```python
from build123d import *

# Parameters (mm, degrees)
F0_W     = 2.5
F0_H     = 84.828298
F0_H_2   = 45.171702
F1_DEPTH = 6
F3_COUNT = 2
F3_ANGLE = 180


with BuildPart() as f1:
    # F0 (on Top) → F1 (new body)
    with BuildSketch(Plane.XY):
        with BuildLine():
            Line((192.326957, -18.864548), (-57.173043, -18.864548))
            Line((-57.173043, -18.864548), (-57.173043, -69.03625))
            ThreePointArc((-57.173043, -69.03625), (-55.427418, -65.103617), (-51.781147, -62.819426))
            Line((-51.781147, -62.819426), (170.496624, -45.052804))
            ThreePointArc((170.496624, -45.052804), (186.918172, -36.548754), (192.326957, -18.864548))
        make_face()
        Polygon((-60.173043, -18.864548), (-57.173043, -18.864548), (-57.173043, 70.96375), (-60.173043, 70.96375), (-60.173043, 65.96375), align=None)
        with Locations((-61.423043, 23.549601)):
            Rectangle(F0_W, F0_H)
        Polygon((-57.173043, -69.03625), (-57.173043, -18.864548), (-60.173043, -18.864548), (-60.173043, -64.03625), (-60.173043, -69.03625), align=None)
        with Locations((-61.423043, -41.450399)):
            Rectangle(F0_W, F0_H_2)
        with BuildLine():
            Line((-57.173043, 70.96375), (-57.173043, -18.864548))
            Line((-57.173043, -18.864548), (192.326957, -18.864548))
            ThreePointArc((192.326957, -18.864548), (191.318788, -13.006753), (188.162474, -7.970102))
            Line((188.162474, -7.970102), (-29.638024, 17.603921))
            Line((-29.638024, 17.603921), (-30.638024, 17.603921))
            Line((-30.638024, 17.603921), (-30.638024, 53.075382))
            Line((-30.638024, 53.075382), (-49.68049, 56.956703))
            ThreePointArc((-49.68049, 56.956703), (-55.182221, 63.02121), (-57.173043, 70.96375))
        make_face()
        with BuildLine():
            Line((-29.638024, 17.603921), (188.162474, -7.970102))
            Line((188.162474, -7.970102), (172.748387, 8.427883))
            ThreePointArc((172.748387, 8.427883), (168.724522, 11.588688), (163.944572, 13.414685))
            Line((163.944572, 13.414685), (-29.638024, 52.871558))
            Line((-29.638024, 52.871558), (-29.638024, 17.603921))
        make_face()
    extrude(amount=F1_DEPTH)

    # F3: F1 ×2 about axis
    f3_axis = Axis((-62.673043, 0.96375, 3), (0, -1, 0))


with BuildPart() as f1_1:
    add(f1.part)
    for i in range(1, F3_COUNT):
        add(f1.part.rotate(f3_axis, i * F3_ANGLE / (F3_COUNT - 1)))


solid = f1_1.part
```
For this review, take the finished solid that the model builds, in its own axes (mm). Coordinates: 2 decimals unless noted, no trailing zeros. Write each loop counter-clockwise with the first axis right and the second up, starting at its lowest first coordinate (ties: lowest second). Pieces come first, ordered by that corner, then holes. Notation, with made-up numbers: (-29, -1.5) -> (14, -1.5) arc R23 ccw to (14, 12.5) -> close; hole circle Ø3 at (85.5, -18.75). An arc over 180 degrees is marked (long way). Put each result on its own line as item: value.
Q1. Wall thickness on L1, parallel to X at y = 8.5, z = 0.5; L2, parallel to Y at x = -1.5, z = 3.25; L3, parallel to Y at x = 44, z = 3.25: over which ranges is each line inside the solid? List them lowest first.
From the geometry:
L1: x = -298.03 to 172.68
L2: y = -58.8 to 47.14
L3: y = -55.16 to 37.86
Q2. Take a section at B-B, the plane x = -122.5. State the section outline as (y, z) points, then the cut area to 3 significant figures.
From the geometry:
outline: (-58.91, 0) -> (47.41, 0) -> (47.41, 6) -> (-58.91, 6) -> close
area: 638 mm2
Q3. Take a section at C-C, the plane y = 1.5. State the section outline as (x, z) points.
From the geometry:
outline: (-304.61, 0) -> (179.26, 0) -> (179.26, 6) -> (-304.61, 6) -> close
Q4. Clearance check with flat-ended pins moving along their axes: pin 1 Ø1 at (x, z) = (-43, 1) entering from +Y; pin 2 Ø1.5 at (x, z) = (-62.5, 3.5) entering from -Y; pin 3 Ø2.5 at (y, z) = (-67.5, 3) entering from -X. State where each tip first meets the part, or that it passes through.
From the geometry:
pin 1: stops at y = 55.7
pin 2: stops at y = -64.04
pin 3: stops at x = -69.1
